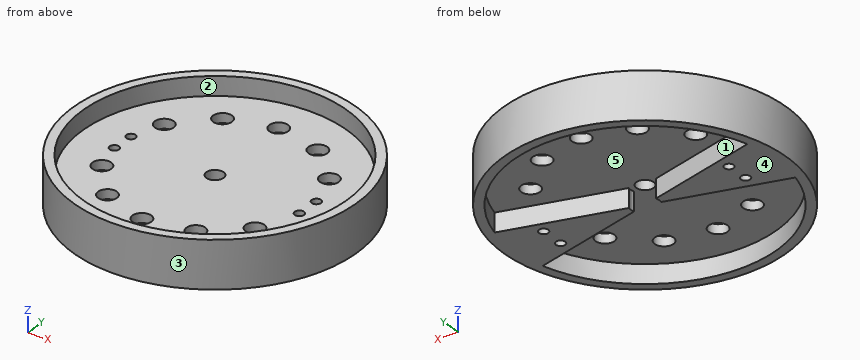
```python
from build123d import *

# Parameters (mm, degrees)
SKETCH1_R               = 38.1
BOSS_EXTRUDE2_DEPTH     = 12.7
SKETCH3_R               = 35.56
CUT_EXTRUDE2_DEPTH      = 5.08
CUT_EXTRUDE3_START      = -5.08
SKETCH4_R               = 35.56
CUT_EXTRUDE3_DEPTH      = 5.08
BOSS_EXTRUDE3_DEPTH     = 5.08
BOSS_EXTRUDE4_DEPTH     = 5.08
SKETCH9_R               = 2.54
CUT_EXTRUDE5_DEPTH      = 55.417684625
CIRPATTERN1_COUNT       = 5
CIRPATTERN1_ANGLE       = 120
SKETCH10_R              = 2.54
CUT_EXTRUDE6_DEPTH      = 55.417684625
CIRPATTERN2_COUNT       = 5
CIRPATTERN2_ANGLE       = 120
CUT_EXTRUDE7_DEPTH      = 55.417684625
CUT_EXTRUDE7_DEPTH_BACK = 55.417684625
SKETCH11_R              = 1.27
CUT_EXTRUDE8_DEPTH      = 55.417684625
CUT_EXTRUDE8_DEPTH_BACK = 55.417684625
SKETCH12_R              = 2.31672553


with BuildPart() as part:
    # Sketch1 → Boss-Extrude2 (new body)
    with BuildSketch(Plane.XY):
        Circle(SKETCH1_R)
    extrude(amount=-BOSS_EXTRUDE2_DEPTH)

    # Sketch3 → Cut-Extrude2 (cut)
    with BuildSketch(Plane.XY):
        Circle(SKETCH3_R)
    extrude(amount=-CUT_EXTRUDE2_DEPTH, mode=Mode.SUBTRACT)

    # Sketch4 → Cut-Extrude3 (cut)
    with BuildSketch(Plane(origin=(0, 0, -12.7), x_dir=(-1, 0, 0), z_dir=(0, 0, -1)).offset(CUT_EXTRUDE3_START)):
        with Locations(Location((0, 0, 0), (0, 0, 180))):
            Circle(SKETCH4_R)
    extrude(amount=CUT_EXTRUDE3_DEPTH, mode=Mode.SUBTRACT)

    # Sketch6 → Boss-Extrude3 (add)
    with BuildSketch(Plane(origin=(0, 0, -7.62), x_dir=(-1, 0, 0), z_dir=(0, 0, -1))):
        with BuildLine():
            Line((-3.81, 0), (-35.56, 0))
            ThreePointArc((-35.56, 0), (-35.25577927, -4.641511395), (-34.348322383, -9.203605244))
            Line((-34.348322383, -9.203605244), (-3.680177398, -0.986100562))
            ThreePointArc((-3.680177398, -0.986100562), (-3.777404922, -0.497304792), (-3.81, 0))
        make_face()
    boss_extrude3 = extrude(amount=BOSS_EXTRUDE3_DEPTH)

    # Mirror2: Boss-Extrude3 across plane
    add(boss_extrude3.mirror(Plane(origin=(3.81, 0, -45.881763645), x_dir=(0, 0, 1), z_dir=(0, -1, 0))))

    # Sketch8 → Boss-Extrude4 (add)
    with BuildSketch(Plane(origin=(0, 0, -7.62), x_dir=(-1, 0, 0), z_dir=(0, 0, -1))):
        with BuildLine():
            Line((3.81, 0), (35.56, 0))
            ThreePointArc((35.56, 0), (35.25577927, -4.641511395), (34.348322383, -9.203605244))
            Line((34.348322383, -9.203605244), (3.680177398, -0.986100562))
            ThreePointArc((3.680177398, -0.986100562), (3.777404922, -0.497304792), (3.81, 0))
        make_face()
    boss_extrude4 = extrude(amount=BOSS_EXTRUDE4_DEPTH)

    # Mirror3: Boss-Extrude4 across plane
    add(boss_extrude4.mirror(Plane(origin=(-3.81, 0, -45.881763645), x_dir=(0, 0, 1), z_dir=(0, -1, 0))))

    # Sketch9 → Cut-Extrude5 (cut, symmetric)
    with BuildSketch(Plane(origin=(0, 0, -7.62), x_dir=(-1, 0, 0), z_dir=(0, 0, -1))):
        with Locations((22.346538839, 12.074444166)):
            Circle(SKETCH9_R)
    cut_extrude5 = extrude(amount=CUT_EXTRUDE5_DEPTH, both=True, mode=Mode.SUBTRACT)

    # CirPattern1: Cut-Extrude5 ×5 about axis
    cirpattern1_axis = Axis((0, 0, 0), (0, 0, -1))
    for i in range(1, CIRPATTERN1_COUNT):
        add(cut_extrude5.rotate(cirpattern1_axis, i * CIRPATTERN1_ANGLE / (CIRPATTERN1_COUNT - 1)), mode=Mode.SUBTRACT)

    # Sketch10 → Cut-Extrude6 (cut, symmetric)
    with BuildSketch(Plane(origin=(0, 0, -7.62), x_dir=(-1, 0, 0), z_dir=(0, 0, -1))):
        with Locations((22.86059693, -11.070370726)):
            Circle(SKETCH10_R)
    cut_extrude6 = extrude(amount=CUT_EXTRUDE6_DEPTH, both=True, mode=Mode.SUBTRACT)

    # CirPattern2: Cut-Extrude6 ×5 about axis
    cirpattern2_axis = Axis((0, 0, 0), (0, 0, 1))
    for i in range(1, CIRPATTERN2_COUNT):
        add(cut_extrude6.rotate(cirpattern2_axis, i * CIRPATTERN2_ANGLE / (CIRPATTERN2_COUNT - 1)), mode=Mode.SUBTRACT)

    # Sketch11 → Cut-Extrude7 (cut, two sides: drawn at the far end of the back side and taken through both)
    with BuildSketch(Plane(origin=(0, 0, -7.62), x_dir=(-1, 0, 0), z_dir=(0, 0, -1)).offset(-CUT_EXTRUDE7_DEPTH_BACK)):
        with Locations((-25.180527268, 3.331823302)):
            Circle(SKETCH11_R)
        with Locations((-25.198683581, -3.191605521)):
            Circle(SKETCH11_R)
        with Locations((25.180527268, 3.331823302)):
            Circle(SKETCH11_R)
        with Locations((25.229521307, -2.937899696)):
            Circle(SKETCH11_R)
    extrude(amount=CUT_EXTRUDE7_DEPTH + CUT_EXTRUDE7_DEPTH_BACK, mode=Mode.SUBTRACT)

    # Sketch12 → Cut-Extrude8 (cut, two sides: drawn at the far end of the back side and taken through both)
    with BuildSketch(Plane(origin=(0, 0, -7.62), x_dir=(-1, 0, 0), z_dir=(0, 0, -1)).offset(-CUT_EXTRUDE8_DEPTH_BACK)):
        Circle(SKETCH12_R)
    extrude(amount=CUT_EXTRUDE8_DEPTH + CUT_EXTRUDE8_DEPTH_BACK, mode=Mode.SUBTRACT)


solid = part.part
```
Check sheet for the modelled part. Datum: model origin and axes. Units: mm. Face numbers are marked on the shaded views. A direction names the side the tool comes from. Give positions to 0.01 mm unless a question says otherwise; leave off trailing zeros. Loops run counter-clockwise (first coordinate to the right, second up) from the corner with the lowest first, then second, coordinate; pieces in that order, holes last. Notation, with made-up numbers: (-16, 37.5) - (41, 37.5) arc R22 ccw to (41, 75.5) - close; hole circle Ø9 at (0.25, 31). An arc over 180 degrees is marked (long way). One line per question, with ' | ' between items. Start each with the question number.
1. Cross-section at A-A, the plane x = -22. Enter the section's corners in (y, z).
2. Cross-section at B-B, the plane z = -3.75. Enter the section's corners in (x, y), plus the area to 3 significant figures.
3. Gauge pin test, flat ends, axial feed: pin 1 Ø5.5 at (x, y) = (0, 0) entering from +Z; pin 2 Ø5 at (y, z) = (-30, -5) entering from -X; pin 3 Ø4 at (y, z) = (11, -6) entering from -X. Record the tip position at first contact, or that the pin passes through.
4. Cross-section at D-D, the plane y = -31.5. Enter the section's corners in (x, z), plus the area to 3 significant figures.
5. Draft check along Y on the marked faces 3, 4 and 5. Enter one of: released by +Y, released by -Y, zero draft, split by the parting line, or undercut.
6. Material ranges on line 1 along Y through (x, z) = (-6, -12); line 2 along Y through (x, z) = (-22.5, -8.5); line 3 along Y through (x, z) = (0, -3.4), recorded low to high. Write a range as [from, to].
7. Cross-section at C-C, the plane z = -9. Enter the section's corners in (x, y).
8. Set-up check for the marked faces 1 and 2: record each of +Z, -Z, +X, -X, +Y, -Y from which the full face is reachable in a straight line by a thin tool's end or side.
Check result:
1) outline: (-31.11, -12.7) - (-27.94, -12.7) - (-27.94, -7.62) - (-13.46, -7.62) - (-13.46, -5.08) - (-27.94, -5.08) - (-27.94, 0) - (-31.11, 0) - close; (-8.68, -7.62) - (-5.89, -7.62) - (-5.89, -12.7) - (5.89, -12.7) - (5.89, -7.62) - (9.56, -7.62) - (9.56, -5.08) - (-8.68, -5.08) - close; (14.59, -7.62) - (27.94, -7.62) - (27.94, -12.7) - (31.11, -12.7) - (31.11, 0) - (27.94, 0) - (27.94, -5.08) - (14.59, -5.08) - close
2) outline: circle Ø76.2 at (0, 0); hole circle Ø71.12 at (0, 0) | area: 588 mm2
3) pin 1: stops at z = -5.08 | pin 2: stops at x = -26.37 | pin 3: stops at x = -37.02
4) outline: (-21.43, -12.7) - (-16.5, -12.7) - (-16.5, -7.62) - (16.5, -7.62) - (16.5, -12.7) - (21.43, -12.7) - (21.43, 0) - (16.5, 0) - (16.5, -5.08) - (-16.5, -5.08) - (-16.5, 0) - (-21.43, 0) - close | area: 209 mm2
5) face 3: split by the parting line | face 4: zero draft | face 5: undercut
6) line 1: y = [-37.62, -35.05], [-1.61, 1.61], [35.05, 37.62] | line 2: y = [-30.75, -27.54], [-6.03, 6.03], [27.54, 30.75] | line 3: y = [-38.1, -35.56], [35.56, 38.1]
7) outline: circle Ø76.2 at (0, 0); hole (-34.35, -9.2) arc R35.56 ccw to (34.35, -9.2) - (3.68, -0.99) arc R3.81 ccw to (3.68, 0.99) - (34.35, 9.2) arc R35.56 ccw to (-34.35, 9.2) - (-3.68, 0.99) arc R3.81 ccw to (-3.68, -0.99) - close; hole circle Ø2.54 at (-25.23, -2.94); hole circle Ø2.54 at (-25.18, 3.33); hole circle Ø2.54 at (25.18, 3.33); hole circle Ø2.54 at (25.2, -3.19)
8) face 1: -Z | face 2: +Z
